from build123d import *

# Parameters (mm, degrees)
BOSS_EXTRUDE1_DEPTH = 2.54
SKETCH1_4_R         = 1.5875
BOSS_EXTRUDE3_DEPTH = 2.9718
SKETCH4_W           = 6.35
SKETCH4_H           = 6.35
BOSS_EXTRUDE4_DEPTH = 6.35
SKETCH5_R           = 1.5875
CUT_EXTRUDE1_DEPTH  = 6.35
FILLET1_R           = 3.175


with BuildPart() as part:
    # Sketch1 → Boss-Extrude1 (new body)
    with BuildSketch(Plane(origin=(0, 0, 0), x_dir=(1, 0, 0), z_dir=(0, 1, 0))):
        with BuildLine():
            Line((-12.7, 3.175), (12.7, 3.175))
            ThreePointArc((12.7, 3.175), (15.875, 0), (12.7, -3.175))
            Line((12.7, -3.175), (-12.7, -3.175))
            ThreePointArc((-12.7, -3.175), (-15.875, 0), (-12.7, 3.175))
        make_face()
    extrude(amount=BOSS_EXTRUDE1_DEPTH)

    # Sketch1<4> → Boss-Extrude3 (add)
    with BuildSketch(Plane(origin=(0, 0, 0), x_dir=(1, 0, 0), z_dir=(0, 1, 0))):
        with Locations(Location((-12.7, 0, 0), (0, 0, 270))):
            Circle(SKETCH1_4_R)
        with Locations(Location((12.7, 0, 0), (0, 0, 270))):
            Circle(SKETCH1_4_R)
    extrude(amount=-BOSS_EXTRUDE3_DEPTH)

    # Sketch4 → Boss-Extrude4 (add)
    with BuildSketch(Plane.XZ):
        Rectangle(SKETCH4_W, SKETCH4_H)
    extrude(amount=BOSS_EXTRUDE4_DEPTH)

    # Sketch5 → Cut-Extrude1 (cut)
    with BuildSketch(Plane(origin=(3.175, 0, 0), x_dir=(0, 0, -1), z_dir=(1, 0, 0))):
        with Locations((0, -3.175)):
            Circle(SKETCH5_R)
    extrude(amount=-CUT_EXTRUDE1_DEPTH, mode=Mode.SUBTRACT)

    # Fillet1
    fillet1_edges = [part.edges().sort_by_distance(p)[0] for p in [
        (0, -6.35, 3.175),
        (0, -6.35, -3.175),
    ]]
    fillet(fillet1_edges, radius=FILLET1_R - 0.0001)  # a hair under: the kernel refuses the full size


solid = part.part
Verification items for the finished model (mm, model axes). A direction names the side the tool comes from. Give positions to 0.01 mm unless a question says otherwise; leave off trailing zeros. Order: outer loops, then holes, each group sorted by start corner. A loop starts at its lowest first (then second) coordinate and runs counter-clockwise, first axis right, second up. Notation, with made-up numbers: M 0.25,-20.5 L 9.25,-20.5 A11 cw 9.25,-1.5 Z; hole C 86.25,-3 d6. An arc over 180 degrees is marked long. Use one line per item in the form item = value. Start each with the question number.
Q1. Section check B-B (y = -2). Enter the section's corners in (x, z) (1 decimal), then the cut area to 3 significant figures.
Q2. Go/stop test with flat-tipped pins: pin 1 Ø3 at (y, z) = (-3.175, 0) entering from +X; pin 2 Ø1.6 at (x, z) = (-12, 0.5) entering from -Y; pin 3 Ø1.9 at (x, z) = (-7.5, 0.5) entering from -Y. Record where each tip stops, or that it passes through.
Q3. Scan lines: line 1 along Y through (x, z) = (2, 0); line 2 along X through (y, z) = (-2, 2) (3 decimals); line 3 along Y through (x, z) = (12.5, -2). Record each from-to range of solid material in increasing order. Write a range as [from, to].
Q4. Mould release check, pull along X, two halves, no side actions. Record for faces 6 (the cylindrical face through (15.874, 1.252, -0.07)), 7 (the flat face through (13, -2.972, 0)), 8 (the cylindrical face through (-15.874, 1.252, 0.07)), 9 (the cylindrical face through (14.274, -1.465, -0.207)): +X half, -X half, draft (parallel to the pull), parting line (faces both ways), or undercut.
Q5. Section check A-A (y = -3.5). Enter the section's corners in (x, z) (3 decimals).
Q6. Section check D-D (x = -5). Enter the section's corners in (y, z) (3 decimals).
Q7. Section check C-C (x = 13). Enter the section's corners in (y, z), then the cut area to 3 significant figures.
Q8. Access from +Z, -Z, +X, -X, +Y, -Y to the whole of each face (thin tool, end or side, straight path). Record for faces 1 (the cylindrical face through (0.044, -4.725, 0.344)), 2 (the flat face through (3.175, -1.7, 1.4)), 3 (the flat face through (0, 0, 3.175)), 4 (the cylindrical face through (-11.126, -1.465, -0.207)), 5 (the cylindrical face through (0.044, -5.445, 2.22)).
Evaluation:
q1.outline = C -12.7,0 d3.2; M -3.2,-3.2 L 3.2,-3.2 L 3.2,-1.1 L -3.2,-1.1 Z; M -3.2,1.1 L 3.2,1.1 L 3.2,3.2 L -3.2,3.2 Z; C 12.7,0 d3.2
q1.area = 42.6 mm2
q2.pin_1 = 14.29
q2.pin_2 = -2.97
q2.pin_3 = 0
q3.line_1 = [-6.35, -4.76], [-1.59, 2.54]
q3.line_2 = [-3.175, 3.175]
q3.line_3 = [0, 2.54]
q4.face_6 = +X half
q4.face_7 = draft
q4.face_8 = -X half
q4.face_9 = undercut
q5.outline = M -3.175,-3.158 L 3.175,-3.158 L 3.175,-1.554 L -3.175,-1.554 Z; M -3.175,1.554 L 3.175,1.554 L 3.175,3.158 L -3.175,3.158 Z
q6.outline = M 0,-3.175 L 2.54,-3.175 L 2.54,3.175 L 0,3.175 Z
q7.outline = M -2.97,-1.56 L 0,-1.56 L 0,-3.16 L 2.54,-3.16 L 2.54,3.16 L 0,3.16 L 0,1.56 L -2.97,1.56 Z
q7.area = 25.3 mm2
q8.face_1 = none
q8.face_2 = +Z, -Z, -Y
q8.face_3 = +Z, +X, -X, +Y, -Y
q8.face_4 = -Y
q8.face_5 = +Z, +X, -X, -Y
